Autodesk Inventor part; units mm, degrees
ref_plane "YZ Plane" through (0, 0, 0) normal (1, 0, 0) x (0, 1, 0)
ref_plane "XZ Plane" through (0, 0, 0) normal (0, 1, 0) x (-1, 0, 0)
ref_plane "XY Plane" through (0, 0, 0) normal (0, 0, 1) x (1, 0, 0)
sketch "Sketch1" plane through (0, 0, 0) normal (0, 0, 1) x (1, 0, 0)
  arc A0 (18.957, 15.5204) -> (15.8526, 18.6801) centre (0, 0) ccw construction
  line L0 (-24.5, 24.5) -> (27, 24.5) construction
  line L1 (27, 24.5) -> (27, -27) construction
  line L2 (27, -27) -> (-24.5, -27) construction
  line L3 (-24.5, -27) -> (-24.5, 24.5) construction
  line L4 (7, -27) -> (27, -27)
  line L5 (27, -27) -> (27, -7)
  arc A1 (27, -7) -> (20.52, 13.4631) centre (-8.55, -7) ccw
  line L6 (7, -27) -> (7, -23.4787)
  line L7 (21.5, 19) -> (0, 0) construction
  line L8 (-21.5, -19) -> (0, 0) construction
  arc A2 (18.8773, 16.6823) -> (23.8177, 16.3773) centre (21.5, 19) ccw construction
  arc A3 (-23.8177, -16.3773) -> (-19.1823, -21.6227) centre (-21.5, -19) ccw
  line L9 (-23.8177, -16.3773) -> (-20.488, -13.4348)
  line L10 (-19.1823, -21.6227) -> (-15.8526, -18.6801)
  line L11 (23.8177, 16.3773) -> (20.52, 13.4631)
  line L12 (19.1823, 21.6227) -> (15.8526, 18.6801)
  arc A4 (7, -23.4787) -> (18.957, 15.5204) centre (0, 0) ccw construction
  arc A5 (15.8526, 18.6801) -> (-20.488, -13.4348) centre (0, 0) ccw
  arc A6 (20.52, 13.4631) -> (18.957, 15.5204) centre (-8.55, -7) ccw construction
  arc A7 (19.1823, 21.6227) -> (18.8773, 16.6823) centre (21.5, 19) ccw construction
  arc A8 (23.8177, 16.3773) -> (19.1823, 21.6227) centre (21.5, 19) ccw
  arc A9 (-18.8773, -16.6823) -> (-23.8177, -16.3773) centre (-21.5, -19) ccw construction
  arc A10 (-19.1823, -21.6227) -> (-18.8773, -16.6823) centre (-21.5, -19) ccw construction
  arc A11 (-15.8526, -18.6801) -> (7, -23.4787) centre (0, 0) ccw
  arc A12 (-20.488, -13.4348) -> (-15.8526, -18.6801) centre (0, 0) ccw construction
  dimension "d0" = 49
  dimension "d1" = 51.5
  dimension "d2" = 51.5
  dimension "d3" = 20
  dimension "d4" = 20
  dimension "d5" = 43
  dimension "d6" = 38
  dimension "d7" = 7
  dimension "d8" = 7
extrude "Extrusion1" add sketch "Sketch1" against normal blind 15
sketch "Sketch2" plane through (7, -27, 0) normal (0, -1, 0) x (1, 0, 0)
  line L0 (20, 0) -> (0, 0)
  line L1 (0, 0) -> (0, -15)
  line L2 (20, -15) -> (0, -15)
  line L3 (20, 0) -> (20, -15)
  line L4 (1.5, -1.5) -> (18.5, -1.5)
  line L5 (18.5, -1.5) -> (18.5, -13.5)
  line L6 (18.5, -13.5) -> (1.5, -13.5)
  line L7 (1.5, -13.5) -> (1.5, -1.5)
  point P0 (-7, 0)
  dimension "d22" = 1.5
extrude "Extrusion2" cut sketch "Sketch2" against normal blind 25 contours L4 L5 L6 L7
hole "Hole1" at (-21.5, -19, 0) at (21.5, 19, 0) direction (0, 0, -1) diameter 4.4 end through all
sketch "Sketch3" plane through (0, 0, -15) normal (0, 0, -1) x (-1, 0, 0)
  arc A0 (20.488, -13.4348) -> (-15.8526, 18.6801) centre (0, 0) ccw
  circle A1 centre (0, 0) radius 18.3084
  circle A2 centre (0, 0) radius 11.7236
extrude "Extrusion3" cut sketch "Sketch3" against normal blind 13.5
properties part number "fan" material "Acetal Resin, Black"
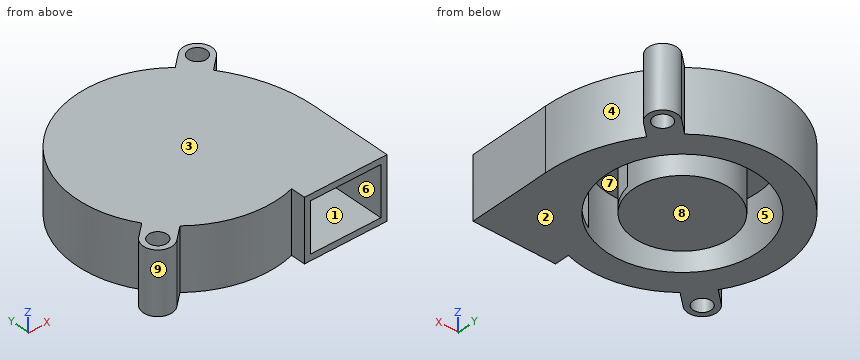
Geometry check sheet. Reference: the model listing, model coordinates, mm. Face numbers are marked on the shaded views. A direction names the side the tool comes from. Coordinates: 2 decimals unless noted, no trailing zeros. Order: outer loops, then holes, each group sorted by start corner. A loop starts at its lowest first (then second) coordinate and runs counter-clockwise, first axis right, second up. Notation, with made-up numbers: M -38.5,-34.5 L -4.5,-34.5 A30 cw -4.5,-3.5 Z; hole C 69,0 d5. An arc over 180 degrees is marked long. Answer as a JSON object with one key per item and string values.
Q1. Tool access check on the marked faces 1, 2, 3, 4 and 5. Record the directions out of +Z, -Z, +X, -X, +Y, -Y that give a thin tool (end or side, any length) a straight path to the whole face; none if there is none.
Results are:
{"face 1": "-Y", "face 2": "-Z, +X, -X, +Y, -Y", "face 3": "+Z, +X, -X, +Y, -Y", "face 4": "+Z, -Z, +X", "face 5": "-Z"}
Q2. Scan lines: line 1 (Y direction, x = 0, z = -8); line 2 (X direction, y = -0.5, z = -2); line 3 (X direction, y = -19, z = -6.75). Record each from-to range of solid material in increasing order.
Results are:
{"line 1": "y = -24.5 to -18.31, -11.72 to 11.72, 18.31 to 24.5", "line 2": "x = -24.49 to -18.3, -11.71 to 11.71, 18.3 to 26.4", "line 3": "x = -25 to -23.7, -19.3 to -16.21, -15.47 to 8.5, 25.5 to 27"}
Q3. Cross-section at A-A on z = -7.5. Record the cut outline in (x, y), and give its area (3 significant figures).
Results are:
{"outline": "M -23.82,-16.38 A3.5 ccw -19.18,-21.62 L -15.85,-18.68 A24.5 ccw 7,-23.48 L 7,-27 L 8.5,-27 L 8.5,-16.22 A18.31 cw long 18.2,-2 L 25.5,-2 L 25.5,-27 L 27,-27 L 27,-7 A35.55 ccw 20.52,13.46 L 23.82,16.38 A3.5 ccw 19.18,21.62 L 15.85,18.68 A24.5 ccw -20.49,-13.43 Z; M 8.5,-8.07 L 8.5,-2 L 11.55,-2 A11.72 ccw long Z; hole C -21.5,-19 d4.4; hole C 21.5,19 d4.4", "area": "1,240 mm²"}
Q4. Release check for a two-part mould opening along Z. For the marked faces 6, 7, 8 and 9 record: released by +Z, released by -Z, zero draft, split by the parting line, or undercut.
Results are:
{"face 6": "undercut", "face 7": "undercut", "face 8": "released by -Z", "face 9": "zero draft"}
Q5. Cross-section at D-D on y = -3. Record the cut outline in (x, z), and give its area (3 significant figures).
Results are:
{"outline": "M -24.32,-15 L -18.06,-15 L -18.06,-1.5 L -11.33,-1.5 L -11.33,-15 L 11.33,-15 L 11.33,-13.5 L 8.5,-13.5 L 8.5,-1.5 L 25.5,-1.5 L 25.5,-13.5 L 18.06,-13.5 L 18.06,-15 L 26.77,-15 L 26.77,0 L -24.32,0 Z", "area": "461 mm²"}
Q6. Depth check by flat-ended pin: pin 1 Ø4 at (x, z) = (-4.5, -8) entering from +Y; pin 2 Ø3 at (x, z) = (12, -5.5) entering from +Y; pin 3 Ø3 at (x, z) = (10.5, -4.5) entering from -Y. Enter the tip coordinate at first touch or a pass-through.
Results are:
{"pin 1": "stops at y = 24.37", "pin 2": "stops at y = 22.14", "pin 3": "stops at y = -2"}
Q7. Cross-section at B-B on x = -21.5. Record the cut outline in (y, z).
Results are:
{"outline": "M -22.5,-15 L -21.2,-15 L -21.2,0 L -22.5,0 Z; M -16.8,-15 L -14.33,-15 L -14.33,0 L -16.8,0 Z; M -11.75,-15 L 11.75,-15 L 11.75,0 L -11.75,0 Z"}
Q8. Cross-section at C-C on x = 17. Record the cut outline in (y, z).
Results are:
{"outline": "M -27,-15 L -6.8,-15 L -6.8,-13.5 L -27,-13.5 Z; M -27,-1.5 L 6.8,-1.5 L 6.8,-15 L 19.69,-15 L 19.69,0 L -27,0 Z"}
